```python
from build123d import *

# Parameters (mm, degrees)
F0_R     = 12.7
F1_DEPTH = 16
F3_D     = 3
F5_DEPTH = 11
F6_R     = 4
F7_DEPTH = 3


with BuildPart() as f1:
    # F0 (on Top) → F1 (new body)
    with BuildSketch(Plane.XY):
        Circle(F0_R)
    extrude(amount=F1_DEPTH)

    # F3 (through all)
    with Locations(Plane.XY.offset(16)):
        with Locations((-8.909959, -3.295851), (1.600689, 9.364176), (7.30927, -6.068325)):
            Hole(F3_D / 2)

    # F4 (on face) → F5 (cut)
    with BuildSketch(Plane.XY.offset(16)):
        Polygon((3.616691, -0.600319), (2.328237, 2.831986), (-1.288454, 3.432305), (-3.616691, 0.600319), (-2.328237, -2.831986), (1.288454, -3.432305), align=None)
    extrude(amount=-F5_DEPTH, mode=Mode.SUBTRACT)

    # F6 (on face) → F7 (join)
    with BuildSketch(Plane(origin=(0, 0, 0), x_dir=(1, 0, 0), z_dir=(0, 0, -1))):
        Circle(F6_R)
    extrude(amount=F7_DEPTH)


solid = f1.part
```
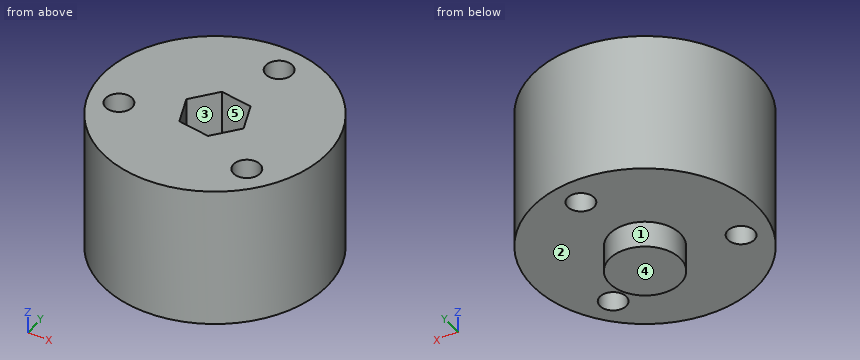
Can you work these out from the model? Positions are in its coordinate system, mm. Face numbers are marked on the shaded views. A direction names the side the tool comes from. Coordinates: 2 decimals unless noted, no trailing zeros. Order: outer loops, then holes, each group sorted by start corner. A loop starts at its lowest first (then second) coordinate and runs counter-clockwise, first axis right, second up.
1. Thinking about a two-plate mould opening in Y: for the marked faces 1, 2 and 3, which applies, +Y half, -Y half, draft (parallel to the pull), parting line (faces both ways), or undercut?
2. I'm going to push flat-ended pins straight in: pin 1 (5 mm diameter, centred on x = 7.31, y = -6.07, fed in from +Z); pin 2 (6 mm diameter, centred on y = -7, z = 8, fed in from -X); pin 3 (1.5 mm diameter, centred on y = -8, z = 7, fed in from -X); pin 4 (2 mm diameter, centred on y = 9, z = 1, fed in from -X). Where does each tip first touch, or does it pass through?
3. I need wall thicknesses on line 1 (X direction, y = -2.75, z = 13); line 2 (Z direction, x = -9.75, y = 0); line 3 (X direction, y = -2.5, z = 12.5). Which ranges of each line are inside material? Lowest first, please.
4. For the marked faces 4 and 5, which set-ups out of +Z, -Z, +X, -X, +Y, -Y let a thin tool reach every point of the face, with its end or its side?
5. If we section it at A-A (z = 8.25): Please give me the cut outline in (x, y).
6. If we section it at B-B (x = -8.5): Please give me the cut outline in (y, z).
7. If we section it at C-C (y = 1.25): Please give me the cut outline in (x, z).
8. If we section it at D-D (z = 0.75): Please give me the cut outline in (x, y), then the cut area to 3 significant figures.
Entries:
1. face 1: parting line
1. face 2: draft
1. face 3: undercut
2. pin 1: stops at z = 16
2. pin 2: stops at x = -12.05
2. pin 3: stops at x = -10.43
2. pin 4: stops at x = -9.86
3. line 1: x = -12.4 to -10.31, -7.51 to -2.36, 1.85 to 12.4
3. line 2: z = 0 to 16
3. line 3: x = -12.45 to -10.18, -7.64 to -2.45, 2.05 to 12.45
4. face 4: -Z, +X, -X, +Y, -Y
4. face 5: +Z
5. outline: circle Ø25.4 at (0, 0); hole circle Ø3 at (-8.91, -3.3); hole (-3.62, 0.6) - (-2.33, -2.83) - (1.29, -3.43) - (3.62, -0.6) - (2.33, 2.83) - (-1.29, 3.43) - close; hole circle Ø3 at (1.6, 9.36); hole circle Ø3 at (7.31, -6.07)
6. outline: (-9.44, 0) - (-4.74, 0) - (-4.74, 16) - (-9.44, 16) - close; (-1.85, 0) - (9.44, 0) - (9.44, 16) - (-1.85, 16) - close
7. outline: (-12.64, 0) - (-3.8, 0) - (-3.8, -3) - (3.8, -3) - (3.8, 0) - (12.64, 0) - (12.64, 16) - (2.92, 16) - (2.92, 5) - (-3.08, 5) - (-3.08, 16) - (-12.64, 16) - close
8. outline: circle Ø25.4 at (0, 0); hole circle Ø3 at (-8.91, -3.3); hole circle Ø3 at (1.6, 9.36); hole circle Ø3 at (7.31, -6.07)
8. area: 486 mm2
